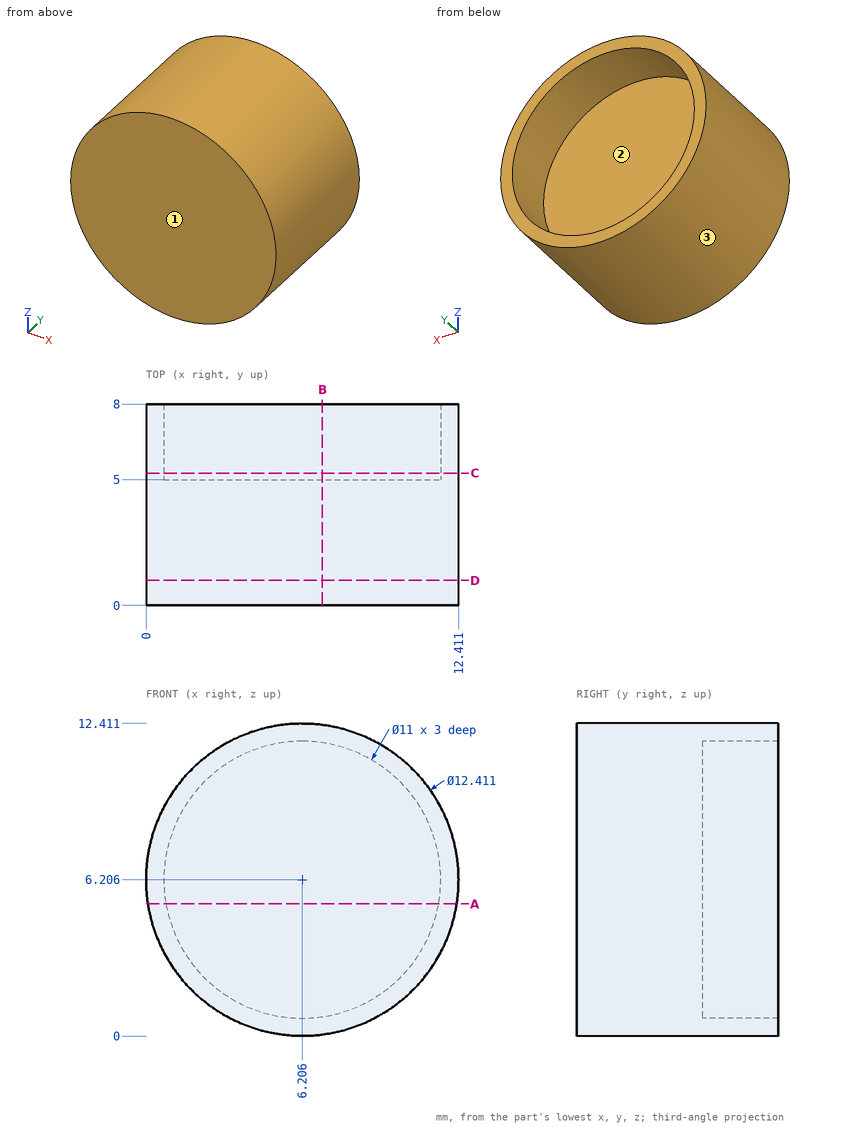
Answer from the drawing. Dimensions are ordinates in mm from the lowest x, y and z of the part. Coordinates: 2 decimals unless noted, no trailing zeros. Loops run counter-clockwise (first coordinate to the right, second up) from the corner with the lowest first, then second, coordinate; pieces in that order, holes last. Notation, with made-up numbers: (87.25, -14.75) - (133.25, -14.75) arc R29 ccw to (133.25, 18.25) - close; hole circle Ø8 at (65, -20). An arc over 180 degrees is marked (long way). Answer in a Markdown table with one row per item.
1. Find section C-C, the plane y = 5.25. Write down the section's boundary in (x, z) (1 decimal).
Conclusion:
| item | result |
|---|---|
| outline | circle Ø12.4 at (6.2, 6.2); hole circle Ø11 at (6.2, 6.2) |
2. Given pin 1 (1.5 mm diameter, centred on y = 2.5, z = 10.5, fed in from +X); pin 2 (1 mm diameter, centred on x = 2, y = 5, fed in from -Z), each flat-ended and moving along its own axis, determine where each tip first touches the part or whether it passes through.
Conclusion:
| item | result |
|---|---|
| pin 1 | stops at x = 11.3 |
| pin 2 | stops at z = 1.23 |
3. Find section A-A, the plane z = 5.25. Write down the section's boundary in (x, y).
Conclusion:
| item | result |
|---|---|
| outline | (0.07, 0) - (12.34, 0) - (12.34, 8) - (11.62, 8) - (11.62, 5) - (0.79, 5) - (0.79, 8) - (0.07, 8) - close |
4. Straight lines are drawn through the part: line 1 (Y direction, x = 7.25, z = 8.25); line 2 (X direction, y = 7.5, z = 6); line 3 (X direction, y = 5.75, z = 7). For each, find the intervals that lie inside material, in ascending order.
Conclusion:
| item | result |
|---|---|
| line 1 | y = 0 to 5 |
| line 2 | x = 0 to 0.71, 11.7 to 12.41 |
| line 3 | x = 0.05 to 0.76, 11.65 to 12.36 |
5. Find section B-B, the plane x = 7. Write down the section's boundary in (y, z).
Conclusion:
| item | result |
|---|---|
| outline | (0, 0.05) - (8, 0.05) - (8, 0.76) - (5, 0.76) - (5, 11.65) - (8, 11.65) - (8, 12.36) - (0, 12.36) - close |
6. Determine the mould class of the marked faces 1, 2 and 3 for opening direction Z: +Z half, -Z half, draft (parallel to the pull), parting line (faces both ways), or undercut.
Conclusion:
| item | result |
|---|---|
| face 1 | draft |
| face 2 | undercut |
| face 3 | parting line |
7. Find section D-D, the plane y = 1. Write down the section's boundary in (x, z) (1 decimal).
Conclusion:
| item | result |
|---|---|
| outline | circle Ø12.4 at (6.2, 6.2) |
